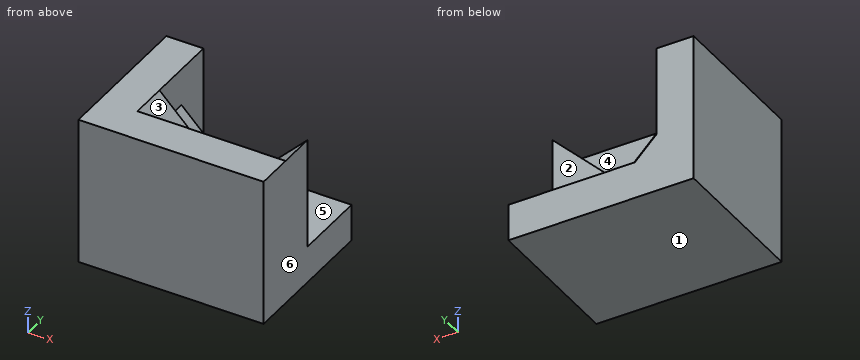
from build123d import *

# Parameters (mm, degrees)
SKETCH1_W           = 50
SKETCH1_H           = 40
BOSS_EXTRUDE1_DEPTH = 40
CUT_EXTRUDE1_DEPTH  = 10
CUT_EXTRUDE2_DEPTH  = 20
CUT_EXTRUDE3_DEPTH  = 10


with BuildPart() as part:
    # Sketch1 → Boss-Extrude1 (new body)
    with BuildSketch(Plane(origin=(0, 0, 0), x_dir=(1, 0, 0), z_dir=(0, 1, 0))):
        with Locations((-15, 0)):
            Rectangle(SKETCH1_W, SKETCH1_H)
    extrude(amount=BOSS_EXTRUDE1_DEPTH)

    # Sketch2 → Cut-Extrude1 (cut)
    with BuildSketch(Plane(origin=(0, 40, 0), x_dir=(1, 0, 0), z_dir=(0, 1, 0))):
        Polygon((-30, -10), (-30, 4.142135624), (-24.142135624, 10), (-10, 10), align=None)
    extrude(amount=-CUT_EXTRUDE1_DEPTH, mode=Mode.SUBTRACT)

    # Sketch3 → Cut-Extrude2 (cut)
    with BuildSketch(Plane(origin=(0, 40, 0), x_dir=(1, 0, 0), z_dir=(0, 1, 0))):
        Polygon((-30, -10), (-30, -20), (10, -20), (10, 10), (-10, 10), align=None)
    extrude(amount=-CUT_EXTRUDE2_DEPTH, mode=Mode.SUBTRACT)

    # Sketch4 → Cut-Extrude3 (cut)
    with BuildSketch(Plane(origin=(0, 20, 0), x_dir=(1, 0, 0), z_dir=(0, 1, 0))):
        Polygon((-30, -20), (-10, 0), (10, -20), align=None)
    extrude(amount=-CUT_EXTRUDE3_DEPTH, mode=Mode.SUBTRACT)


solid = part.part
Read the model definition and answer for the solid it produces. Units are mm, in the model's axes. Face numbers are marked on the shaded views. A direction names the side the tool comes from. Coordinates: 2 decimals unless noted, no trailing zeros. Loops run counter-clockwise (first coordinate to the right, second up) from the corner with the lowest first, then second, coordinate; pieces in that order, holes last. Notation, with made-up numbers: (-30, 72) -> (-15, 72) arc R7 cw to (-15, 82) -> close; hole circle Ø4 at (3.5, -27.5). An arc over 180 degrees is marked (long way). Write item = value, one per line. Start each with the question number.
1) Find the intervals of material crossed by L1, parallel to Y at x = -5.5, z = 2.5; L2, parallel to X at y = 18.5, z = 3; L3, parallel to Y at x = -20.5, z = -4, in increasing order. Write a range as from..to.
2) The mould has two halves that part along X. Classify the marked faces 4, 5 and 6: pulls with the +X half, pulls with the -X half, needs draft (parallel to the pull), parting line crosses it, or undercut.
3) Given P1, Ø6, axis at x = -12.5, z = 14, coming from the +Y side; P2, Ø24, axis at x = -9, z = 3.5, coming from the +Y side; P3, Ø10, axis at x = -10.5, y = 27, coming from the +Z side, each flat-ended and moving along its own axis, determine where each tip first touches the part or whether it passes through.
4) The part is cut by section D-D, the plane x = -17. Determine the outline of the cut face in (y, z).
5) The part is cut by section C-C, the plane z = 5.5. Determine the outline of the cut face in (x, y), plus the area to 4 significant figures.
6) For the marked faces 1, 2 and 3, determine the directions among +Z, -Z, +X, -X, +Y, -Y from which every point of the face is accessible in a straight line to the end or side of a thin tool.
7) The part is cut by section A-A, the plane x = -7.5. Determine the outline of the cut face in (y, z), plus the area to 3 significant figures.
8) The part is cut by section B-B, the plane y = 22.5. Determine the outline of the cut face in (x, z), plus the area to 3 significant figures.
Result:
q1.L1 = 0..20
q1.L2 = -40..-13, -7..10
q1.L3 = 0..30
q2.face_4 = undercut
q2.face_5 = needs draft
q2.face_6 = pulls with the +X half
q3.P1 = 10
q3.P2 = 30
q3.P3 = -4.5
q4.outline = (0, -20) -> (40, -20) -> (40, -10) -> (30, -10) -> (30, -3) -> (20, -3) -> (20, 7) -> (10, 7) -> (10, 20) -> (0, 20) -> close
q5.outline = (-40, 0) -> (10, 0) -> (10, 20) -> (-4.5, 20) -> (-4.5, 10) -> (-15.5, 10) -> (-15.5, 20) -> (-25.5, 20) -> (-25.5, 30) -> (-30, 30) -> (-30, 40) -> (-40, 40) -> close
q5.area = 1,135 mm²
q6.face_1 = -Z, +X, -X, +Y, -Y
q6.face_2 = +Z, +X, +Y
q6.face_3 = +Z, +Y
q7.outline = (0, -20) -> (40, -20) -> (40, -10) -> (20, -10) -> (20, 2.5) -> (10, 2.5) -> (10, 20) -> (0, 20) -> close
q7.area = 825 mm²
q8.outline = (-40, -20) -> (10, -20) -> (10, -10) -> (-10, -10) -> (-30, 10) -> (-30, 20) -> (-40, 20) -> close
q8.area = 1,000 mm²
